Model file for the job. Use its own axes, mm. Round coordinates to 2 decimals unless told otherwise and drop trailing zeros. Write each loop counter-clockwise with the first axis right and the second up, starting at its lowest first coordinate (ties: lowest second). Pieces come first, ordered by that corner, then holes. Notation, with made-up numbers: (-5, 10) - (8, 10) arc R24 ccw to (8, 36) - close; hole circle Ø11 at (41.5, -4.75). An arc over 180 degrees is marked (long way). One line per item, written item: value.
from build123d import *

# Parameters (mm, degrees)
SKETCH_2_R               = 0.75
EXTRUDE_1_DEPTH          = 7
PATTERN_CIRCULAR_1_COUNT = 20


with BuildPart() as part:
    # 草图1 → 旋转1 (revolve)
    with BuildSketch(Plane.XY, mode=Mode.PRIVATE) as revolve_1_sk:
        Polygon((-9, 4.25), (-5, 4.25), (-5, 4), (-2.5, 4), (-2.5, -4), (-5, -4), (-5, -4.25), (-9, -4.25), (-9, -3.25), (-6, -3.25), (-6, 3.25), (-9, 3.25), align=None)
    revolve(revolve_1_sk.sketch.rotate(Axis((0, 36.523336922, 0), (0, -1, 0)), 270), axis=Axis((0, 36.523336922, 0), (0, -1, 0)))

    # 草图2 → 凸台-拉伸1 (add)
    with BuildSketch(Plane(origin=(0, -3.25, 0), x_dir=(1, 0, 0), z_dir=(0, 1, 0))):
        with Locations((3.878999087, -4.577484689)):
            Circle(SKETCH_2_R)
    extrude_1 = extrude(amount=EXTRUDE_1_DEPTH)

    # 阵列(圆周)1: 凸台-拉伸1 ×20 about axis
    pattern_circular_1_axis = Axis((0, 0, 0), (0, 1, 0))
    for i in range(1, PATTERN_CIRCULAR_1_COUNT):
        add(extrude_1.rotate(pattern_circular_1_axis, i * 360 / PATTERN_CIRCULAR_1_COUNT))


solid = part.part
1. Drop flat-ended pins along their axis: pin 1 (1 mm diameter, centred on x = -2.5, y = -2, fed in from +Z); pin 2 (1 mm diameter, centred on y = 1, z = 2.5, fed in from +X); pin 3 (9 mm diameter, centred on x = 0, z = 0, fed in from +Y). Give the stop position or say it passes through.
Report:
pin 1: z = 6.31
pin 2: x = 6.31
pin 3: y = 4
2. Mould opens along X. For faces 1 (the face through (-0.486, -0.046, -6.732)), 2 (the face through (2.44, -0.06, -0.54)), 3 (the face through (4, 4.25, 4)) say: released by +X, released by -X, zero draft, split by the parting line, or undercut.
Report:
face 1: undercut
face 2: undercut
face 3: zero draft
3. Band-saw the part on D-D on y = 3.75. Write the cut outline in (x, z).
Report:
outline: circle Ø18 at (0, 0); hole circle Ø5 at (0, 0)
4. Band-saw the part on B-B on x = 0. Write the cut outline in (y, z).
Report:
outline: (-4.25, -9) - (-3.25, -9) - (-3.25, -6.59) - (3.25, -6.59) - (3.25, -9) - (4.25, -9) - (4.25, -5) - (4, -5) - (4, -2.5) - (-4, -2.5) - (-4, -5) - (-4.25, -5) - close; (-4.25, 5) - (-4, 5) - (-4, 2.5) - (4, 2.5) - (4, 5) - (4.25, 5) - (4.25, 9) - (3.25, 9) - (3.25, 6.59) - (-3.25, 6.59) - (-3.25, 9) - (-4.25, 9) - close
5. Band-saw the part on C-C on z = 0. Write the cut outline in (x, y).
Report:
outline: (-9, -4.25) - (-5, -4.25) - (-5, -4) - (-2.5, -4) - (-2.5, 4) - (-5, 4) - (-5, 4.25) - (-9, 4.25) - (-9, 3.25) - (-6.59, 3.25) - (-6.59, -3.25) - (-9, -3.25) - close; (2.5, -4) - (5, -4) - (5, -4.25) - (9, -4.25) - (9, -3.25) - (6.59, -3.25) - (6.59, 3.25) - (9, 3.25) - (9, 4.25) - (5, 4.25) - (5, 4) - (2.5, 4) - close
6. Band-saw the part on A-A on z = -8. Write the cut outline in (x, y).
Report:
outline: (-4.12, -4.25) - (4.12, -4.25) - (4.12, -3.25) - (-4.12, -3.25) - close; (-4.12, 3.25) - (4.12, 3.25) - (4.12, 4.25) - (-4.12, 4.25) - close
7. Wall check: probe 1 along Y at (x, z) = (-2, 6.75); probe 2 along X at (y, z) = (4.1, 0); probe 3 along X at (y, z) = (-1.5, 0). Give the ranges that are in metal, low to high. Write a range as [from, to].
Report:
probe 1: [-4.25, -3.25], [3.25, 4.25]
probe 2: [-9, -5], [5, 9]
probe 3: [-6.59, -2.5], [2.5, 6.59]
